```python
from build123d import *

# Parameters (mm, degrees)
SKETCH2_W           = 6.35
SKETCH2_H           = 73.66
BOSS_EXTRUDE1_DEPTH = 71.12
CUT_EXTRUDE1_DEPTH  = 71.12
SKETCH4_W           = 1.5875
SKETCH4_H           = 14.422052326
CUT_EXTRUDE2_DEPTH  = 71.12
SKETCH6_W           = 32.023370344
SKETCH6_H           = 8.840748178
SKETCH6_R           = 2.286
BOSS_EXTRUDE2_DEPTH = 3.175
BOSS_EXTRUDE3_DEPTH = 3.175


with BuildPart() as part:
    # Sketch2 → Boss-Extrude1 (new body)
    with BuildSketch(Plane(origin=(0, 0, 0), x_dir=(1, 0, 0), z_dir=(0, 1, 0))):
        with Locations((3.175, -36.83)):
            Rectangle(SKETCH2_W, SKETCH2_H)
    extrude(amount=BOSS_EXTRUDE1_DEPTH)

    # Sketch3 → Cut-Extrude1 (cut)
    with BuildSketch(Plane(origin=(6.35, 0, 0), x_dir=(0, 0, -1), z_dir=(1, 0, 0))):
        with BuildLine():
            ThreePointArc((0, 0), (-42.190194821, 21.385195311), (-73.66, 56.697947674))
            Line((-73.66, 56.697947674), (-73.66, 0))
            Line((-73.66, 0), (0, 0))
        make_face()
        with BuildLine():
            Line((0, 71.12), (-73.66, 71.12))
            ThreePointArc((-73.66, 71.12), (-44.704376489, 30.667054561), (0, 8.840748178))
            Line((0, 8.840748178), (0, 71.12))
        make_face()
    extrude(amount=-CUT_EXTRUDE1_DEPTH, mode=Mode.SUBTRACT)

    # Sketch4 → Cut-Extrude2 (cut)
    with BuildSketch(Plane.XY.offset(73.66)):
        with Locations((2.38125, 63.908973837)):
            Rectangle(SKETCH4_W, SKETCH4_H)
        with Locations((3.96875, 63.908973837)):
            Rectangle(SKETCH4_W, SKETCH4_H)
    extrude(amount=-CUT_EXTRUDE2_DEPTH, mode=Mode.SUBTRACT)

    # Sketch6 → Boss-Extrude2 (add)
    with BuildSketch(Plane(origin=(0, 0, 0), x_dir=(-1, 0, 0), z_dir=(0, 0, -1))):
        with Locations((-3.175, 4.420374089)):
            Rectangle(SKETCH6_W, SKETCH6_H)
        with Locations((-15.875, 4.420374089)):
            Circle(SKETCH6_R, mode=Mode.SUBTRACT)
        with Locations((9.525, 4.420374089)):
            Circle(SKETCH6_R, mode=Mode.SUBTRACT)
    extrude(amount=BOSS_EXTRUDE2_DEPTH)

    # Sketch7 → Boss-Extrude3 (add)
    with BuildSketch(Plane(origin=(1.5875, 0, 0), x_dir=(0, 0, -1), z_dir=(1, 0, 0))):
        Polygon((-73.66, 67.596150372), (-72.201792637, 67.596150372), (-73.66, 71.12), align=None)
    extrude(amount=BOSS_EXTRUDE3_DEPTH)


solid = part.part
```
Could you check a few things on this model? Use its own coordinates, in mm. A direction names the side the tool comes from. Round coordinates to 2 decimals unless told otherwise and drop trailing zeros. Loops run counter-clockwise (first coordinate to the right, second up) from the corner with the lowest first, then second, coordinate; pieces in that order, holes last. Notation, with made-up numbers: (19, -1.75) -> (35, -1.75) arc R8 cw to (35, 13.25) -> close; hole circle Ø4 at (38, 14.25). An arc over 180 degrees is marked (long way). One line per question, with ' | ' between items.
(1) For faces 5 (the face through (4.762, 61, 71)), 6 (the face through (13, 4, 0)), 7 (the face through (-12.837, 4, -2)), 8 (the face through (3, 0, -2)), 9 (the face through (0, 25, 40)), which set-ups out of +Z, -Z, +X, -X, +Y, -Y let a thin tool reach every point of the face, with its end or its side?
Model answer:
face 5: +Z, -Z | face 6: +Z, +X, +Y, -Y | face 7: +Z, -Z, -X, +Y, -Y | face 8: +Z, -Z, +X, -X, -Y | face 9: +Z, -X, +Y, -Y
(2) For pin 1 Ø12 at (x, y) = (3.5, 16.5) entering from +Z; pin 2 Ø2 at (x, z) = (5, 55) entering from +Y; pin 3 Ø1.6 at (x, z) = (3, 70.5) entering from +Y, each with a flat end and sliding along its axis, tell me the tip position at first contact or that it passes through.
Model answer:
pin 1: stops at z = 43.62 | pin 2: stops at y = 41.85 | pin 3: stops at y = 56.7
(3) Thinking about a two-plate mould opening in X: for faces 1 (the face through (1.588, 61, 71)), 2 (the face through (3.22, 20.98, 41.66)), 3 (the face through (13.763, 3.545, -1.565)), 4 (the face through (6.35, 25, 40)), which applies, released by +X, released by -X, zero draft, split by the parting line, or undercut?
Model answer:
face 1: undercut | face 2: zero draft | face 3: undercut | face 4: released by +X
(4) If we section it at B-B on x = 17: List the corners of the cut face in (y, z) for me (3 decimals), and give its area (3 significant figures).
Model answer:
outline: (0, -3.175) -> (2.43, -3.175) -> (2.43, 0) -> (0, 0) -> close; (6.41, -3.175) -> (8.841, -3.175) -> (8.841, 0) -> (6.41, 0) -> close | area: 15.4 mm^2
(5) If we section it at A-A on y = 59.5: List the corners of the cut face in (x, z) for me.
Model answer:
outline: (0, 68.23) -> (1.59, 68.23) -> (1.59, 73.66) -> (0, 73.66) -> close; (4.76, 68.23) -> (6.35, 68.23) -> (6.35, 73.66) -> (4.76, 73.66) -> close
(6) If we section it at D-D on z = 20.5: List the corners of the cut face in (x, y) for me.
Model answer:
outline: (0, 7.92) -> (6.35, 7.92) -> (6.35, 15.47) -> (0, 15.47) -> close
(7) If I drill on probe 1 along X at (y, z) = (9, 17); probe 2 along Z at (x, y) = (10, 5.5) (3 decimals); probe 3 along Z at (x, y) = (2, 46.5), over which ranges is the centre line in solid material (lowest first)?
Model answer:
probe 1: x = 0 to 6.35 | probe 2: z = -3.175 to 0 | probe 3: z = 59.78 to 66.84
(8) If we section it at C-C on x = 12: List the corners of the cut face in (y, z) for me (3 decimals), and give its area (3 significant figures).
Model answer:
outline: (0, -3.175) -> (8.841, -3.175) -> (8.841, 0) -> (0, 0) -> close | area: 28.1 mm^2
